Verification items for the finished model (mm, model axes). Face numbers are marked on the shaded views. A direction names the side the tool comes from. Give positions to 0.01 mm unless a question says otherwise; leave off trailing zeros. Write each loop counter-clockwise with the first axis right and the second up, starting at its lowest first coordinate (ties: lowest second). Pieces come first, ordered by that corner, then holes. Notation, with made-up numbers: (-40, 86) -> (-10, 86) arc R17 ccw to (-10, 93) -> close; hole circle Ø6 at (57, -18). An arc over 180 degrees is marked (long way). Write item = value, one per line.
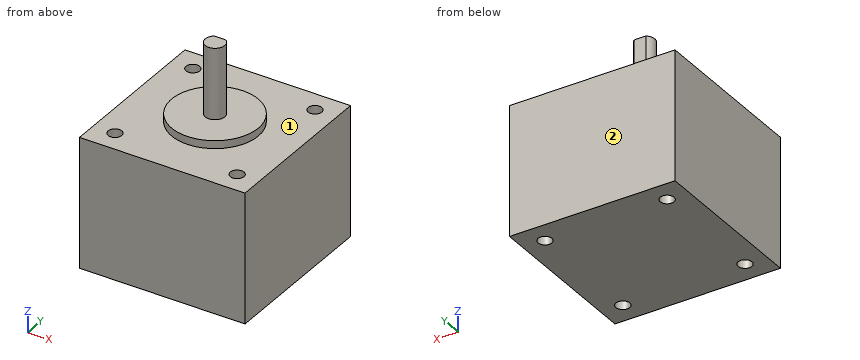
Autodesk Inventor part; units mm, degrees
ref_plane "YZ Plane" through (0, 0, 0) normal (1, 0, 0) x (0, 1, 0)
ref_plane "XZ Plane" through (0, 0, 0) normal (0, 1, 0) x (-1, 0, 0)
ref_plane "XY Plane" through (0, 0, 0) normal (0, 0, 1) x (1, 0, 0)
sketch "Sketch1" plane through (0, 0, 0) normal (0, 0, 1) x (1, 0, 0)
  circle A0 centre (0, 0) radius 2.5
  line L0 (-15.5, 15.5) -> (15.5, 15.5) construction
  line L1 (15.5, 15.5) -> (15.5, -15.5) construction
  line L2 (15.5, -15.5) -> (-15.5, -15.5) construction
  line L3 (-15.5, -15.5) -> (-15.5, 15.5) construction
  line L4 (-15.5, 15.5) -> (15.5, -15.5) construction
  circle A1 centre (-15.5, 15.5) radius 1.75
  circle A2 centre (15.5, 15.5) radius 1.75
  circle A3 centre (15.5, -15.5) radius 1.75
  circle A4 centre (-15.5, -15.5) radius 1.75
  line L5 (-21, 21) -> (21, 21)
  line L6 (21, 21) -> (21, -21)
  line L7 (21, -21) -> (-21, -21)
  line L8 (-21, -21) -> (-21, 21)
  line L9 (-21, -21) -> (21, 21) construction
  dimension "d0" = 5
  dimension "d1" = 31
  dimension "d2" = 3.5
  dimension "d3" = 42
extrude "Extrusion1" add sketch "Sketch1" against normal blind 33 contours A0 | L5 L6 L7 L8
extrude "Extrusion2" add sketch "Sketch1" along normal blind 20 contours A0
sketch "Sketch2" plane through (0, 0, 0) normal (0, 0, 1) x (1, 0, 0)
  circle A0 centre (0, 0) radius 11
  dimension "d8" = 22
extrude "Extrusion3" add sketch "Sketch2" along normal blind 2
sketch "Sketch3" plane through (0, 0, 20) normal (0, 0, 1) x (1, 0, 0)
  circle A0 centre (0, 0) radius 2.5
  line L0 (-1.5, 2) -> (1.5, 2)
  circle A1 centre (0, 0) radius 2.5
  arc A2 (1.5, 2) -> (-1.5, 2) centre (0, 0) ccw
  dimension "d11" = 4.5
extrude "Extrusion4" cut sketch "Sketch3" against normal up to surface (18 mm away) contours L0 A0 picked at (-0.3466, 2.0912)
sketch "Sketch4" plane through (0, 0, 0) normal (0, 0, 1) x (1, 0, 0)
  circle A0 centre (-15.5, 15.5) radius 1.75
  circle A1 centre (-15.5, 15.5) radius 3
  circle A2 centre (15.5, 15.5) radius 1.75
  circle A3 centre (15.5, 15.5) radius 3
  point P0 (0, 0)
  dimension "d14" = 6
  dimension "d15" = 6
properties part number "stepper"
Item 1: Set-up check for the marked faces 1 and 2: record each of +Z, -Z, +X, -X, +Y, -Y from which the full face is reachable in a straight line by a thin tool's end or side.
Response values:
face_1 = +Z
face_2 = +Z, -Z, +X, -X, +Y
Item 2: Sectioned sample at C-C on z = -12. Record the cut outline in (x, y).
Response values:
outline = (-21, -21) -> (21, -21) -> (21, 21) -> (-21, 21) -> close; hole circle Ø3.5 at (-15.5, -15.5); hole circle Ø3.5 at (-15.5, 15.5); hole circle Ø3.5 at (15.5, -15.5); hole circle Ø3.5 at (15.5, 15.5)
Item 3: Sectioned sample at A-A on x = 15.5. Record the cut outline in (y, z).
Response values:
outline = (-21, -33) -> (-17.25, -33) -> (-17.25, 0) -> (-21, 0) -> close; (-13.75, -33) -> (13.75, -33) -> (13.75, 0) -> (-13.75, 0) -> close; (17.25, -33) -> (21, -33) -> (21, 0) -> (17.25, 0) -> close
Item 4: Sectioned sample at D-D on y = 0. Record the cut outline in (x, z).
Response values:
outline = (-21, -33) -> (21, -33) -> (21, 0) -> (11, 0) -> (11, 2) -> (2.5, 2) -> (2.5, 20) -> (-2.5, 20) -> (-2.5, 2) -> (-11, 2) -> (-11, 0) -> (-21, 0) -> close
Item 5: Material ranges on line 1 (Y direction, x = -15.5, z = -8); line 2 (X direction, y = 15, z = -21); line 3 (Z direction, x = 14, y = -10), recorded low to high.
Response values:
line_1 = -21 to -17.25, -13.75 to 13.75, 17.25 to 21
line_2 = -21 to -17.18, -13.82 to 13.82, 17.18 to 21
line_3 = -33 to 0
Item 6: Go/stop test with flat-tipped pins: P1, Ø12, axis at x = -11.5, z = 13, coming from the +Y side; P2, Ø5.5, axis at x = 15.5, y = -15.5, coming from the -Z side; P3, Ø1.5, axis at x = 0, z = 14.5, coming from the +Y side; P4, Ø5, axis at x = 2.5, y = 16, coming from the +Z side. Record where each tip stops, or that it passes through.
Response values:
P1 = through
P2 = -33
P3 = 2
P4 = 0
